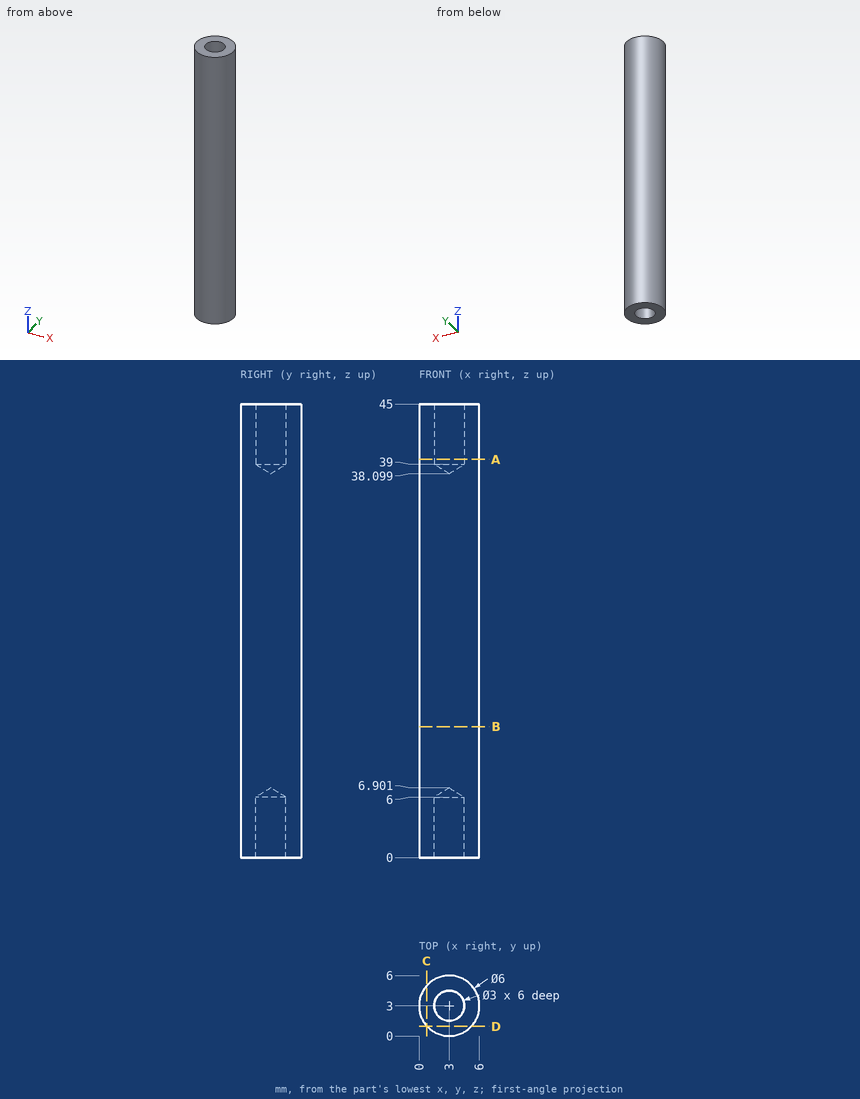
Geometry check sheet. Reference: drawing and pictorial views, mm from the part's lowest x, y, z. Give positions to 0.01 mm unless a question says otherwise; leave off trailing zeros. Order: outer loops, then holes, each group sorted by start corner. A loop starts at its lowest first (then second) coordinate and runs counter-clockwise, first axis right, second up. Notation, with made-up numbers: (5, 2) -> (44, 2) arc R28 cw to (44, 21) -> close; hole circle Ø9 at (66.5, 78.5). An arc over 180 degrees is marked (long way). Use CSV: the item, a comma, the result in double quotes. Start each with the question number.
1) Material ranges on line 1 (Y direction, x = 3, z = 41); line 2 (X direction, y = 3.1, z = 12); line 3 (X direction, y = 4.7, z = 10), recorded low to high. Write a range as from..to.
2) Sectioned sample at B-B, the plane z = 13. Record the boundary of the cut face in (x, y), plus the area to 3 significant figures.
3) Sectioned sample at C-C, the plane x = 0.75. Record the boundary of the cut face in (y, z).
4) Sectioned sample at A-A, the plane z = 39.5. Record the boundary of the cut face in (x, y), plus the area to 3 significant figures.
5) Go/stop test with flat-tipped pins: P1, Ø3.5, axis at x = 3, y = 3, coming from the -Z side; P2, Ø1.5, axis at y = 1, z = 19.5, coming from the -X side; P3, Ø2.5, axis at x = 3, y = 3, coming from the -Z side; P4, Ø1.5, axis at x = 2, z = 29, coming from the +Y side. Record where each tip stops, or that it passes through.
6) Sectioned sample at D-D, the plane y = 0.95. Record the boundary of the cut face in (x, z).
Recorded:
1,line 1,"0..1.5, 4.5..6"
1,line 2,"0..6"
1,line 3,"0.53..5.47"
2,outline,"circle Ø6 at (3, 3)"
2,area,"28.3 mm2"
3,outline,"(1.02, 0) -> (4.98, 0) -> (4.98, 45) -> (1.02, 45) -> close"
4,outline,"circle Ø6 at (3, 3); hole circle Ø3 at (3, 3)"
4,area,"21.2 mm2"
5,P1,"z = 0"
5,P2,"x = 0.27"
5,P3,"z = 6.15"
5,P4,"y = 5.99"
6,outline,"(0.81, 0) -> (5.19, 0) -> (5.19, 45) -> (0.81, 45) -> close"
